Could you check a few things on this model? Use its own coordinates, in mm. Round coordinates to 2 decimals unless told otherwise and drop trailing zeros. Loops run counter-clockwise (first coordinate to the right, second up) from the corner with the lowest first, then second, coordinate; pieces in that order, holes last. Notation, with made-up numbers: (75, 79.25) - (117, 79.25) arc R25 cw to (117, 115.25) - close; hole circle Ø5 at (77, -20). An arc over 180 degrees is marked (long way). Use one line per item in the form item = value.
```python
from build123d import *

# Parameters (mm, degrees)
SKETCH1_W           = 30
SKETCH1_H           = 70
BOSS_EXTRUDE1_DEPTH = 3
SKETCH2_R           = 1.5
SKETCH2_W           = 21
SKETCH2_H           = 45
CUT_EXTRUDE1_DEPTH  = 39.19685851


with BuildPart() as part:
    # Sketch1 → Boss-Extrude1 (new body)
    with BuildSketch(Plane(origin=(0, 0, 0), x_dir=(0, 0, -1), z_dir=(1, 0, 0))):
        Rectangle(SKETCH1_W, SKETCH1_H)
    extrude(amount=BOSS_EXTRUDE1_DEPTH)

    # Sketch2 → Cut-Extrude1 (cut, through all)
    with BuildSketch(Plane(origin=(3, 0, 0), x_dir=(0, 0, -1), z_dir=(1, 0, 0))):
        with Locations((0, 28.5)):
            Circle(SKETCH2_R)
        with Locations(Location((0, -28.5, 0), (0, 0, 180))):
            Circle(SKETCH2_R)
        Rectangle(SKETCH2_W, SKETCH2_H)
    extrude(amount=-CUT_EXTRUDE1_DEPTH, mode=Mode.SUBTRACT)


solid = part.part
```
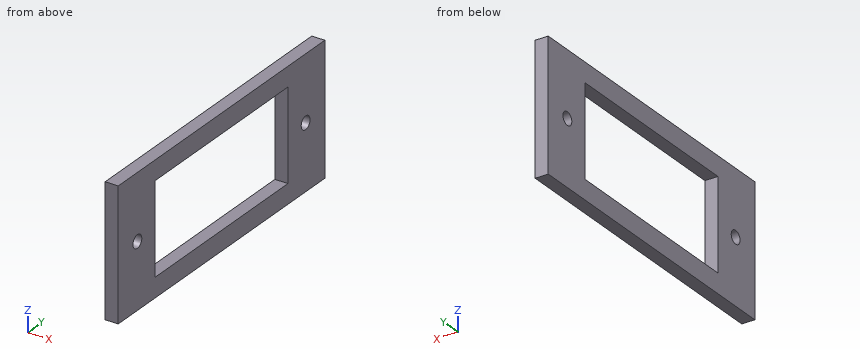
1. For P1, Ø2.5, axis at y = -28.5, z = 0, coming from the -X side (3 decimals), with a flat end and sliding along its axis, tell me the tip position at first contact or that it passes through.
Solution:
P1 = through
2. Please list where these lines run through material, in increasing order: line 1 along Y through (x, z) = (2.3, 0); line 2 along Y through (x, z) = (1, -10.25); line 3 along Z through (x, y) = (2.7, -28.5).
Solution:
line_1 = -35 to -30, -27 to -22.5, 22.5 to 27, 30 to 35
line_2 = -35 to -22.5, 22.5 to 35
line_3 = -15 to -1.5, 1.5 to 15
3. If we section it at A-A, the plane z = -2.25: Write out the boundary of the cut face in (x, y), plus the area to 3 significant figures.
Solution:
outline = (0, -35) - (3, -35) - (3, -22.5) - (0, -22.5) - close; (0, 22.5) - (3, 22.5) - (3, 35) - (0, 35) - close
area = 75.0 mm^2
4. If we section it at C-C, the plane x = 1.2: Write out the boundary of the cut face in (y, z), plus the area to 3 significant figures.
Solution:
outline = (-35, -15) - (35, -15) - (35, 15) - (-35, 15) - close; hole circle Ø3 at (-28.5, 0); hole (-22.5, -10.5) - (22.5, -10.5) - (22.5, 10.5) - (-22.5, 10.5) - close; hole circle Ø3 at (28.5, 0)
area = 1,140 mm^2
5. If we section it at B-B, the plane y = 10: Write out the boundary of the cut face in (x, z), plus the area to 3 significant figures.
Solution:
outline = (0, -15) - (3, -15) - (3, -10.5) - (0, -10.5) - close; (0, 10.5) - (3, 10.5) - (3, 15) - (0, 15) - close
area = 27.0 mm^2
